Here's the drawing with two shaded views (mm, measured from the low corner). I have some questions. A direction names the side the tool comes from. Give positions to 0.01 mm unless a question says otherwise; leave off trailing zeros. Use one line per item in the form item = value. Start each with the question number.
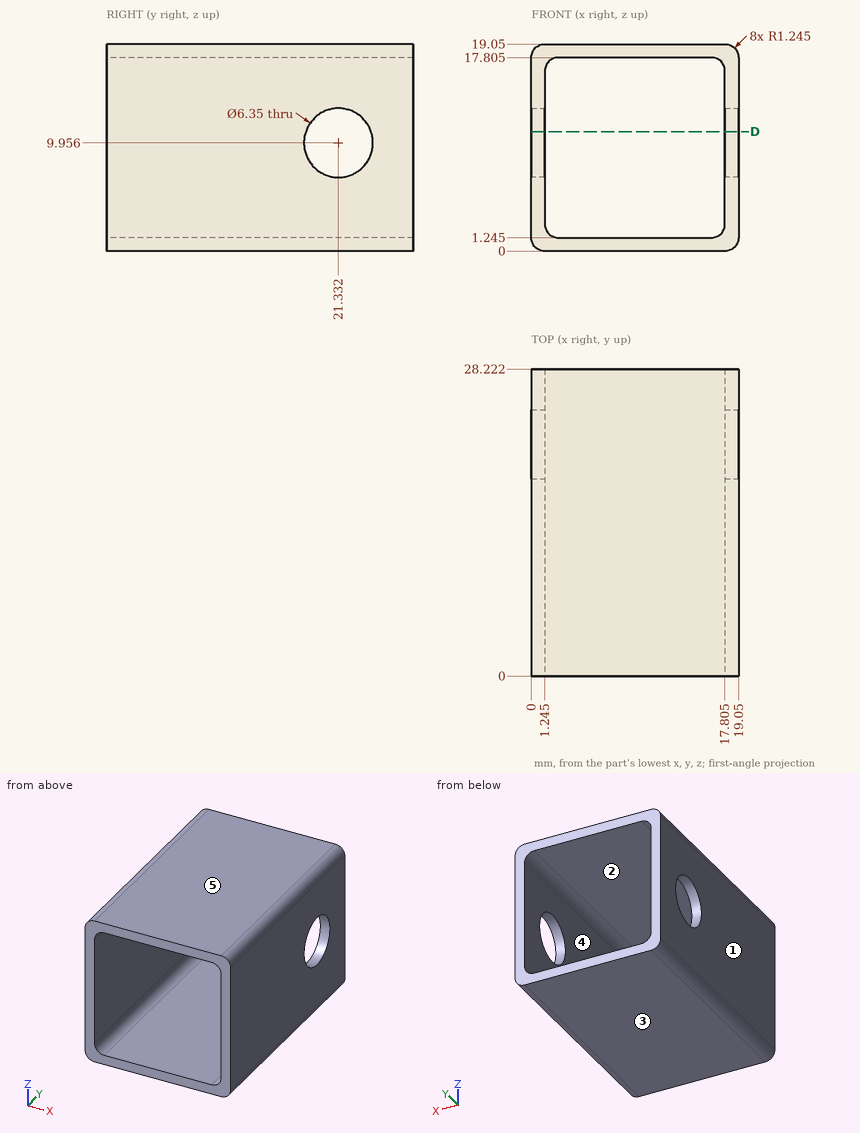
1. We'd pull the mould along Z, two halves only. Please class the marked faces 1, 2 and 3: pulls with the +Z half, pulls with the -Z half, needs draft (parallel to the pull), parting line crosses it, or undercut.
2. I want a section at D-D, the plane z = 11. Give the number of separate pieces and of enclosed holes in the cut face.
3. For P1, Ø6, axis at y = 19, z = 6, coming from the -X side, with a flat end and sliding along its axis, tell me the tip position at first contact or that it passes through.
4. Please list where these lines run through material, in increasing order: line 1 (X direction, y = 7.25, z = 16.75); line 2 (Z direction, x = 1, y = 15) (1 decimal).
5. For the marked faces 4 and 5, which set-ups out of +Z, -Z, +X, -X, +Y, -Y let a thin tool reach every point of the face, with its end or its side?
Result sheet:
q1.face_1 = needs draft
q1.face_2 = undercut
q1.face_3 = pulls with the -Z half
q2.separate_pieces = 4
q2.enclosed_holes = 0
q3.P1 = 0
q4.line_1 = 0 to 1.26, 17.79 to 19.05
q4.line_2 = 0 to 19
q5.face_4 = +Y, -Y
q5.face_5 = +Z, +X, -X, +Y, -Y
